Could you check a few things on this model? Use its own coordinates, in mm. A direction names the side the tool comes from. Round coordinates to 2 decimals unless told otherwise and drop trailing zeros. Loops run counter-clockwise (first coordinate to the right, second up) from the corner with the lowest first, then second, coordinate; pieces in that order, holes last. Notation, with made-up numbers: (70.5, 4.5) -> (121.5, 4.5) arc R22 cw to (121.5, 28.5) -> close; hole circle Ø6 at (44, 83.5). An arc over 180 degrees is marked (long way). Put each result on its own line as item: value. Start each with the question number.
1. If we mould it in two halves opening along Y, with no side actions, what happens to faces 5 (the flat face through (-13, 33, 4)), 6 (the cylindrical face through (-34.408, -18.934, 1.232))? For each: pulls with the +Y half, pulls with the -Y half, needs draft (parallel to the pull), parting line crosses it, or undercut.
2. Imagine slicing it at D-D, the plane x = -15. Please give me the cut outline in (y, z), and give its area (3 significant figures).
3. Imagine slicing it at A-A, the plane y = 0. Please give me the cut outline in (x, z), and give its area (3 significant figures).
4. I'm going to push flat-ended pins straight in: P1, Ø11, axis at x = 15, y = 25.98, coming from the -Z side; P2, Ø22.5, axis at x = -15, y = 25.98, coming from the +Z side; P3, Ø2, axis at y = 17, z = 2, coming from the -X side; P4, Ø2, axis at y = -18, z = 1.5, coming from the +X side. Where does each tip first touch, or does it pass through?
5. I need wall thicknesses on line 1 (Y direction, x = 0, z = 1.25); line 2 (X direction, y = 29.5, z = 3.45); line 3 (Y direction, x = 15, z = 1.6). Which ranges of each line are inside material? Lowest first, please. Write a range as [from, to].
6. Imagine slicing it at B-B, the plane x = 0. Please give me the cut outline in (y, z).
7. Imagine slicing it at C-C, the plane x = -30. Please give me the cut outline in (y, z), and give its area (3 significant figures).
8. Which directions (+Z, -Z, +X, -X, +Y, -Y) give clear straight access to the entire face, cutting with the end or side of a thin tool? Please do faces 1 (the flat face through (-12.762, -7.395, 1.232)), 2 (the flat face through (5, -7, 0)), 3 (the flat face through (27, 16, 1)), 4 (the flat face through (-13, 0, 2.5)).
```python
from build123d import *

# Parameters (mm, degrees)
CYLINDER_R            = 42.75
CYLINDER_DEPTH        = 2.5
CYLINDER001_R         = 12.25
CYLINDER001_DEPTH     = 4
CYLINDER002_R         = 12.25
CYLINDER002_DEPTH     = 4
POLARPATTERN_COUNT    = 6
SKETCH_R              = 7
POCKET_DEPTH          = 4.001
SKETCH001_R           = 7
POCKET001_DEPTH       = 245.963807
POLARPATTERN001_COUNT = 6
SKETCH002_R           = 1.5
POCKET002_DEPTH       = 245.963807
POLARPATTERN002_COUNT = 3
SKETCH003_W           = 3.25
SKETCH003_H           = 6.5
POCKET003_DEPTH       = 245.963807
POLARPATTERN003_COUNT = 6
POCKET004_DEPTH       = 1


with BuildPart() as part:
    # Cylinder → Cylinder (join)
    with BuildSketch(Plane.XY):
        Circle(CYLINDER_R)
    extrude(amount=CYLINDER_DEPTH)

    # Cylinder001 → Cylinder001 (join)
    with BuildSketch(Plane.XY):
        Circle(CYLINDER001_R)
    extrude(amount=CYLINDER001_DEPTH)

    # Cylinder002 → Cylinder002 (join)
    with BuildSketch(Plane(origin=(30, 0, 0), x_dir=(1, 0, 0), z_dir=(0, 0, 1))):
        Circle(CYLINDER002_R)
    cylinder002 = extrude(amount=CYLINDER002_DEPTH)

    # PolarPattern: Cylinder002 ×6 about axis
    polarpattern_axis = Axis((0, 0, 0), (0, 0, 1))
    for i in range(1, POLARPATTERN_COUNT):
        add(cylinder002.rotate(polarpattern_axis, i * 360 / POLARPATTERN_COUNT))

    # Sketch → Pocket (cut, through all)
    with BuildSketch(Plane.XY):
        Circle(SKETCH_R)
    extrude(amount=POCKET_DEPTH, mode=Mode.SUBTRACT)

    # Sketch001 → Pocket001 (cut, through all)
    with BuildSketch(Plane.XY):
        with Locations((-30, 0)):
            Circle(SKETCH001_R)
    pocket001 = extrude(amount=POCKET001_DEPTH, mode=Mode.SUBTRACT)

    # PolarPattern001: Pocket001 ×6 about axis
    polarpattern001_axis = Axis((0, 0, 0), (0, 0, 1))
    for i in range(1, POLARPATTERN001_COUNT):
        add(pocket001.rotate(polarpattern001_axis, i * 360 / POLARPATTERN001_COUNT), mode=Mode.SUBTRACT)

    # Sketch002 → Pocket002 (cut, through all)
    with BuildSketch(Plane.XY):
        with Locations((0, 38)):
            Circle(SKETCH002_R)
    pocket002 = extrude(amount=POCKET002_DEPTH, mode=Mode.SUBTRACT)

    # PolarPattern002: Pocket002 ×3 about axis
    polarpattern002_axis = Axis((0, 0, 0), (0, 0, 1))
    for i in range(1, POLARPATTERN002_COUNT):
        add(pocket002.rotate(polarpattern002_axis, i * 360 / POLARPATTERN002_COUNT), mode=Mode.SUBTRACT)

    # Sketch003 → Pocket003 (cut, through all)
    with BuildSketch(Plane.XY):
        with Locations((0, 18)):
            Rectangle(SKETCH003_W, SKETCH003_H)
    pocket003 = extrude(amount=POCKET003_DEPTH, mode=Mode.SUBTRACT)

    # PolarPattern003: Pocket003 ×6 about axis
    polarpattern003_axis = Axis((0, 0, 0), (0, 0, 1))
    for i in range(1, POLARPATTERN003_COUNT):
        add(pocket003.rotate(polarpattern003_axis, i * 360 / POLARPATTERN003_COUNT), mode=Mode.SUBTRACT)

    # Sketch004 → Pocket004 (cut, symmetric)
    with BuildSketch(Plane(origin=(24, 14, 0), x_dir=(0.5, -0.866025, 0), z_dir=(0, 0, 1))):
        Polygon((0, 0), (1.5, 6), (-1.5, 6), align=None)
    extrude(amount=POCKET004_DEPTH, both=True, mode=Mode.SUBTRACT)


solid = part.part
```
Entries:
1. face 5: needs draft
1. face 6: undercut
2. outline: (-40.03, 0) -> (-32.98, 0) -> (-32.98, 4) -> (-38.23, 4) -> (-38.23, 2.5) -> (-40.03, 2.5) -> close; (-18.98, 0) -> (-10.54, 0) -> (-10.54, 2.5) -> (-13.73, 2.5) -> (-13.73, 4) -> (-18.98, 4) -> close; (-6.78, 0) -> (6.78, 0) -> (6.78, 2.5) -> (-6.78, 2.5) -> close; (10.54, 0) -> (18.98, 0) -> (18.98, 4) -> (13.73, 4) -> (13.73, 2.5) -> (10.54, 2.5) -> close; (32.98, 0) -> (40.03, 0) -> (40.03, 2.5) -> (38.23, 2.5) -> (38.23, 4) -> (32.98, 4) -> close
2. area: 143 mm^2
3. outline: (-42.75, 0) -> (-37, 0) -> (-37, 4) -> (-42.25, 4) -> (-42.25, 2.5) -> (-42.75, 2.5) -> close; (-23, 0) -> (-7, 0) -> (-7, 4) -> (-12.25, 4) -> (-12.25, 2.5) -> (-17.75, 2.5) -> (-17.75, 4) -> (-23, 4) -> close; (7, 0) -> (23, 0) -> (23, 4) -> (17.75, 4) -> (17.75, 2.5) -> (12.25, 2.5) -> (12.25, 4) -> (7, 4) -> close; (37, 0) -> (42.75, 0) -> (42.75, 2.5) -> (42.25, 2.5) -> (42.25, 4) -> (37, 4) -> close
3. area: 156 mm^2
4. P1: through
4. P2: z = 4
4. P3: x = -39.64
4. P4: x = 39.22
5. line 1: [-42.75, -21.25], [-14.75, -7], [7, 14.75], [21.25, 36.5], [39.5, 42.75]
5. line 2: [-26.73, -21.05], [-8.95, -3.27], [3.27, 8.95], [21.05, 26.73]
5. line 3: [-40.03, -32.98], [-18.98, -10.54], [-6.78, 6.78], [10.54, 18.98], [32.98, 40.03]
6. outline: (-42.75, 0) -> (-21.25, 0) -> (-21.25, 2.5) -> (-42.75, 2.5) -> close; (-14.75, 0) -> (-7, 0) -> (-7, 4) -> (-12.25, 4) -> (-12.25, 2.5) -> (-14.75, 2.5) -> close; (7, 0) -> (14.75, 0) -> (14.75, 2.5) -> (12.25, 2.5) -> (12.25, 4) -> (7, 4) -> close; (21.25, 0) -> (36.5, 0) -> (36.5, 2.5) -> (21.25, 2.5) -> close; (39.5, 0) -> (42.75, 0) -> (42.75, 2.5) -> (39.5, 2.5) -> close
7. outline: (-30.46, 0) -> (-7, 0) -> (-7, 4) -> (-12.25, 4) -> (-12.25, 2.5) -> (-30.46, 2.5) -> close; (7, 0) -> (30.46, 0) -> (30.46, 2.5) -> (12.25, 2.5) -> (12.25, 4) -> (7, 4) -> close
7. area: 133 mm^2
8. face 1: +Z, -Z
8. face 2: -Z, +X, -X, +Y, -Y
8. face 3: -Z
8. face 4: +Z
